Here's how the part is built. I have some questions about the finished solid (model axes, mm). Give positions to 0.01 mm unless a question says otherwise; leave off trailing zeros. Loops run counter-clockwise (first coordinate to the right, second up) from the corner with the lowest first, then second, coordinate; pieces in that order, holes last. Notation, with made-up numbers: (55, -32) -> (74, -32) arc R28 cw to (74, -9) -> close; hole circle Ø3 at (-32, 72.5). An arc over 180 degrees is marked (long way). Answer in a Markdown table with one row per item. Add a question column.
Item 1: If I drill on line 1 (Z direction, x = 3.5, y = 1.5); line 2 (Z direction, x = 1.5, y = -2.5); line 3 (Y direction, x = -0.5, z = 0), over which ranges is the centre line in solid material (lowest first)?
Item 2: If we section it at C-C (x = 2.5): Write out the boundary of the cut face in (y, z).
Item 3: If we section it at B-B (y = -1.5): Write out the boundary of the cut face in (x, z).
Item 4: For P1, Ø6, axis at x = -3, y = 4.5, coming from the +Z side; P2, Ø1, axis at y = -3, z = 62.5, coming from the +X side; P3, Ø1.5, axis at y = 2, z = 63.5, coming from the +X side, each with a flat end and sliding along its axis, tell me the tip position at first contact or that it passes through.
Item 5: If we section it at A-A (z = 170): Write out the boundary of the cut face in (x, y), then the cut area to 3 significant figures.
Item 6: If we section it at D-D (z = 14.5): Write out the boundary of the cut face in (x, y), then the cut area to 3 significant figures.
```python
from build123d import *

# Parameters (mm, degrees)
SKETCH3_R           = 5
BOSS_EXTRUDE1_DEPTH = 170
SKETCH4_R           = 6
BOSS_EXTRUDE2_DEPTH = 5
SKETCH5_R           = 4
SKETCH5_R_2         = 3.999944286
CUT_EXTRUDE1_DEPTH  = 12


with BuildPart() as part:
    # Sketch3 → Boss-Extrude1 (new body)
    with BuildSketch(Plane.XY):
        Circle(SKETCH3_R)
    extrude(amount=BOSS_EXTRUDE1_DEPTH)

    # Sketch4 → Boss-Extrude2 (add, symmetric)
    with BuildSketch(Plane(origin=(0, 0, 0), x_dir=(0, 0, -1), z_dir=(1, 0, 0))):
        with Locations((-170, 0)):
            Circle(SKETCH4_R)
        Circle(SKETCH4_R)
    extrude(amount=BOSS_EXTRUDE2_DEPTH, both=True)

    # Sketch5 → Cut-Extrude1 (cut)
    with BuildSketch(Plane(origin=(5, 0, 0), x_dir=(0, 0, -1), z_dir=(1, 0, 0))):
        with Locations((-170, 0)):
            Circle(SKETCH5_R)
        Circle(SKETCH5_R_2)
    extrude(amount=-CUT_EXTRUDE1_DEPTH, mode=Mode.SUBTRACT)


solid = part.part
```
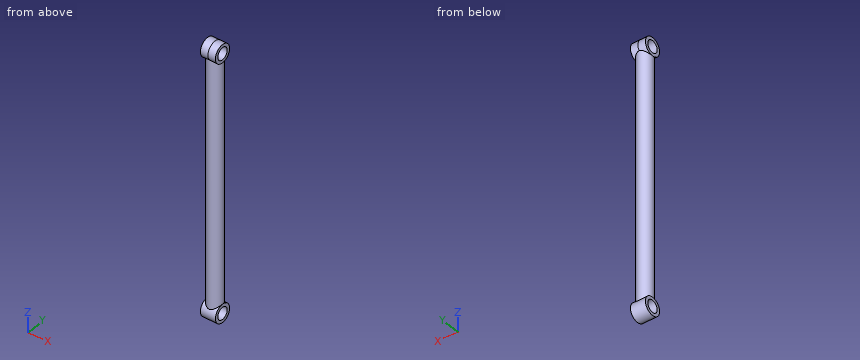
Recorded:
| question | item | result |
|---|---|---|
| 1 | line 1 | z = -5.81 to -3.71, 3.71 to 166.29, 173.71 to 175.81 |
| 1 | line 2 | z = -5.45 to -3.12, 3.12 to 166.88, 173.12 to 175.45 |
| 1 | line 3 | y = -6 to -4, 4 to 6 |
| 2 | outline | (-4.33, 4.15) arc R6 ccw (long way) to (4.33, 4.15) -> (4.33, 165.85) arc R6 ccw (long way) to (-4.33, 165.85) -> close; hole circle Ø8 at (0, 0); hole circle Ø8 at (0, 170) |
| 3 | outline | (-5, -5.81) -> (5, -5.81) -> (5, -3.71) -> (-5, -3.71) -> close; (-5, 3.71) -> (5, 3.71) -> (5, 5.81) -> (4.77, 5.81) -> (4.77, 164.19) -> (5, 164.19) -> (5, 166.29) -> (-5, 166.29) -> (-5, 164.19) -> (-4.77, 164.19) -> (-4.77, 5.81) -> (-5, 5.81) -> close; (-5, 173.71) -> (5, 173.71) -> (5, 175.81) -> (-5, 175.81) -> close |
| 4 | P1 | stops at z = 175.81 |
| 4 | P2 | stops at x = 4.33 |
| 4 | P3 | stops at x = 4.84 |
| 5 | outline | (-5, -6) -> (5, -6) -> (5, -4) -> (-5, -4) -> close; (-5, 4) -> (5, 4) -> (5, 6) -> (-5, 6) -> close |
| 5 | area | 40.0 mm^2 |
| 6 | outline | circle Ø10 at (0, 0) |
| 6 | area | 78.5 mm^2 |
